Verification items for the finished model (mm, model axes). Face numbers are marked on the shaded views. A direction names the side the tool comes from. Give positions to 0.01 mm unless a question says otherwise; leave off trailing zeros. Loops run counter-clockwise (first coordinate to the right, second up) from the corner with the lowest first, then second, coordinate; pieces in that order, holes last. Notation, with made-up numbers: (71.25, 50.25) -> (75.25, 50.25) arc R13 ccw to (75.25, 64.25) -> close; hole circle Ø1 at (-29.5, 21). An arc over 180 degrees is marked (long way). Answer in a Markdown table with one row per item. Add a question column.
Q1. Material ranges on probe 1 along Y at (x, z) = (69.5, 17); probe 2 along X at (y, z) = (-265.5, 59); probe 3 along X at (y, z) = (21, 5), recorded low to high.
Q2. Set-up check for the marked faces 1, 2 and 3: record each of +Z, -Z, +X, -X, +Y, -Y from which the full face is reachable in a straight line by a thin tool's end or side.
Q3. Section check D-D on x = -189. Give the number of separate pieces and of enclosed holes in the cut face, and give its area (3 significant figures).
Q4. Gauge pin test, flat ends, axial feed: P1, Ø10, axis at x = -161.5, z = -57.5, coming from the -Y side; P2, Ø20.5, axis at y = 95.5, z = 32, coming from the +X side; P3, Ø6, axis at x = 124.5, z = 67.5, coming from the -Y side. Record the tip position at first contact, or that the pin passes through.
Q5. Section check B-B on z = 38. Enter the section's corners in (x, y), and give its area (3 significant figures).
Q6. Release check for a two-part mould opening along X. For the marked faces 4 and 5 record: pulls with the +X half, pulls with the -X half, needs draft (parallel to the pull), parting line crosses it, or undercut.
Q7. Section check C-C on y = 5.5. Enter the section's corners in (x, z), and give its area (3 significant figures).
```python
from build123d import *

# Parameters (mm, degrees)
SKETCH1_W           = 400
SKETCH1_H           = 600
BOSS_EXTRUDE1_DEPTH = 89.5
SKETCH2_W           = 315
SKETCH2_H           = 350
CUT_EXTRUDE1_DEPTH  = 1.5
SKETCH3_W           = 18.5
SKETCH3_H           = 3.1
CUT_EXTRUDE2_DEPTH  = 600
SKETCH5_W           = 3.1
SKETCH5_H           = 18.5
CUT_EXTRUDE3_DEPTH  = 363
BOSS_EXTRUDE2_DEPTH = 400


with BuildPart() as part:
    # Sketch1 → Boss-Extrude1 (new body)
    with BuildSketch(Plane.XY):
        Rectangle(SKETCH1_W, SKETCH1_H)
    extrude(amount=BOSS_EXTRUDE1_DEPTH)

    # Sketch2 → Cut-Extrude1 (cut)
    with BuildSketch(Plane.XY.offset(89.5)):
        with Locations((0, 68.5)):
            Rectangle(SKETCH2_W, SKETCH2_H)
    extrude(amount=-CUT_EXTRUDE1_DEPTH, mode=Mode.SUBTRACT)

    # Sketch3 → Cut-Extrude2 (cut)
    with BuildSketch(Plane.XZ.offset(300)):
        with Locations((-190.75, 70.55)):
            Rectangle(SKETCH3_W, SKETCH3_H)
    cut_extrude2 = extrude(amount=-CUT_EXTRUDE2_DEPTH, mode=Mode.SUBTRACT)

    # Mirror1: Cut-Extrude2 across plane
    add(cut_extrude2.mirror(Plane(origin=(0, 0, 0), x_dir=(0, 0, 1), z_dir=(1, 0, 0))), mode=Mode.SUBTRACT)

    # Sketch5 → Cut-Extrude3 (cut)
    with BuildSketch(Plane(origin=(181.5, 0, 0), x_dir=(0, 0, -1), z_dir=(1, 0, 0))):
        with Locations((-70.55, -290.75)):
            Rectangle(SKETCH5_W, SKETCH5_H)
    cut_extrude3 = extrude(amount=-CUT_EXTRUDE3_DEPTH, mode=Mode.SUBTRACT)

    # Mirror2: Cut-Extrude3 across plane
    add(cut_extrude3.mirror(Plane.ZX), mode=Mode.SUBTRACT)

    # Sketch12 → Boss-Extrude2 (add)
    with BuildSketch(Plane.ZY.offset(200)):
        Polygon((-55.28029253, -151.145910296), (-91, -193.715), (-91, -249.285), (-55.28029253, -291.854089704), (-9.082539564, -300), (0, -300), (0, -141.398503221), align=None)
    extrude(amount=-BOSS_EXTRUDE2_DEPTH)

    # Sweep1: sweep along a path in Sketch11
    with BuildLine(Plane.XY) as sweep1_path:
        Line((-200, -35), (-200, -378))
        ThreePointArc((-200, -378), (-194.142135624, -392.142135624), (-180, -398))
        Line((-180, -398), (180, -398))
        ThreePointArc((180, -398), (194.142135624, -392.142135624), (200, -378))
        Line((200, -378), (200, -35))
    # Sketch10 → Sweep1 (sweep)
    with BuildSketch(Plane(origin=(0, -35, 0), x_dir=(1, 0, 0), z_dir=(0, 1, 0))):
        with BuildLine():
            Line((-200, 0.5), (-200, -61.5))
            ThreePointArc((-200, -61.5), (-200.585786438, -62.914213562), (-202, -63.5))
            Line((-202, -63.5), (-222.5, -63.5))
            Line((-222.5, -63.5), (-222.5, -60.5))
            Line((-222.5, -60.5), (-205, -60.5))
            ThreePointArc((-205, -60.5), (-203.585786438, -59.914213562), (-203, -58.5))
            Line((-203, -58.5), (-203, -2.5))
            ThreePointArc((-203, -2.5), (-203.585786438, -1.085786438), (-205, -0.5))
            Line((-205, -0.5), (-222.5, -0.5))
            Line((-222.5, -0.5), (-222.5, 2.5))
            Line((-222.5, 2.5), (-202, 2.5))
            ThreePointArc((-202, 2.5), (-200.585786438, 1.914213562), (-200, 0.5))
        make_face()
    sweep(path=sweep1_path.line)


solid = part.part
```
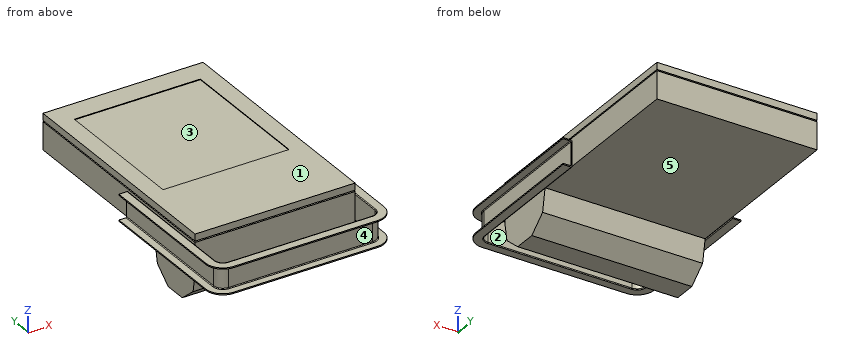
Taken from the geometry:
| question | item | result |
|---|---|---|
| 1 | probe 1 | y = -401 to -398, -300 to 300 |
| 1 | probe 2 | x = -203.06 to 203.06 |
| 1 | probe 3 | x = -200 to 200 |
| 2 | face 1 | +Z, +X, -X, +Y, -Y |
| 2 | face 2 | +Z, -Z |
| 2 | face 3 | +Z |
| 3 | separate pieces | 3 |
| 3 | enclosed holes | 0 |
| 3 | area | 64,000 mm² |
| 4 | P1 | stops at y = -292.34 |
| 4 | P2 | stops at x = 200 |
| 4 | P3 | stops at y = -300 |
| 5 | outline | (-203, -378) arc R23 ccw to (-180, -401) -> (180, -401) arc R23 ccw to (203, -378) -> (203, -35) -> (200, -35) -> (200, 300) -> (-200, 300) -> (-200, -35) -> (-203, -35) -> close; hole (-200, -378) arc R20 ccw to (-180, -398) -> (180, -398) arc R20 ccw to (200, -378) -> (200, -300) -> (-200, -300) -> close |
| 5 | area | 243,000 mm² |
| 6 | face 4 | needs draft |
| 6 | face 5 | undercut |
| 7 | outline | (-200, 0) -> (200, 0) -> (200, 69) -> (181.5, 69) -> (181.5, 72.1) -> (200, 72.1) -> (200, 89.5) -> (157.5, 89.5) -> (157.5, 88) -> (-157.5, 88) -> (-157.5, 89.5) -> (-200, 89.5) -> (-200, 72.1) -> (-181.5, 72.1) -> (-181.5, 69) -> (-200, 69) -> close |
| 7 | area | 35,200 mm² |
